Solid Edge part; units mm, degrees
sketch "Sketch1" plane through (0, 0, 0) normal (1, 0, 0) x (0, 1, 0)
  line L0 (0, 0) -> (0, 3.175)
  line L1 (22.225, 3.175) -> (0, 3.175)
  line L2 (22.225, 25.4) -> (22.225, 3.175)
  line L3 (22.225, 25.4) -> (25.4, 25.4)
  line L4 (25.4, 25.4) -> (25.4, 0)
  line L5 (25.4, 0) -> (0, 0)
  dimension "D1" = 25.4
  dimension "D2" = 25.4
extrude "Protrusion1" add sketch "Sketch1" along normal blind 50.8
sketch "Sketch2" plane through (25.4, 12.7, 0) normal (0, 0, -1) x (-1, 0, 0)
  line L0 (-22.225, -1.778) -> (-22.225, 7.874)
  line L1 (-22.225, 7.874) -> (22.225, 7.874)
  line L2 (22.225, 7.874) -> (22.225, -1.778)
  line L3 (22.225, -1.778) -> (-22.225, -1.778)
  dimension "D1" = 22.225
extrude "Cutout1" cut sketch "Sketch2" against normal through all
fillet "Round_1" radius 3.175 4 edges at (3.175, 10.922, 1.5875) (47.625, 10.922, 1.5875) (47.625, 20.574, 1.5875) (3.175, 20.574, 1.5875)
sketch "Sketch3" plane through (25.4, 25.4, 12.7) normal (0, 1, 0) x (1, 0, 0)
  line L0 (-25.4, -12.7) -> (-25.4, 0)
  line L1 (-25.4, 0) -> (25.4, 0)
  line L2 (25.4, 0) -> (25.4, -12.7)
  line L3 (25.4, -12.7) -> (-25.4, -12.7)
  dimension "D1" = 25.4
extrude "Cutout2" cut sketch "Sketch3" against normal through all
hole "Hole_1" at (42.8625, 25.4, 6.35) direction (0, -1, 0) diameter 3.9675 end up to next
hole "Hole1" at (7.9375, 25.4, 6.35) direction (0, -1, 0) diameter 3.9675 end up to next
sketch "Sketch4" plane through (25.4, 12.7, 0) normal (0, 0, -1) x (-1, 0, 0)
  line L0 (-25.4, -12.7) -> (-25.4, -4.953)
  line L1 (-25.4, -4.953) -> (25.4, -4.953)
  line L2 (25.4, -4.953) -> (25.4, -12.7)
  line L3 (25.4, -12.7) -> (-25.4, -12.7)
  dimension "D1" = 25.4
extrude "Cutout3" cut sketch "Sketch4" against normal through all
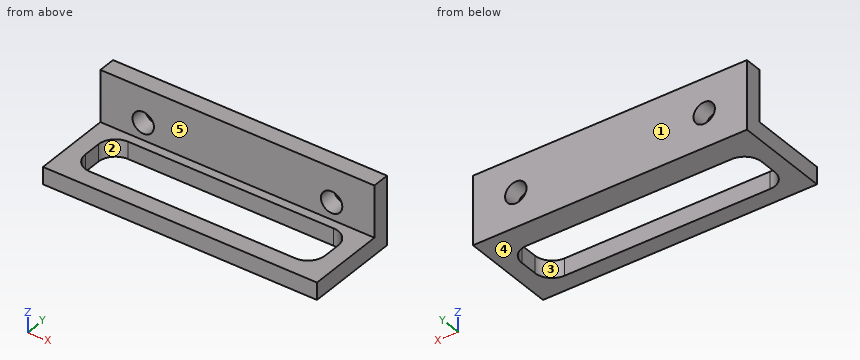
Work out the finished part from the listing and answer in its coordinate system (mm). Face numbers are marked on the shaded views. A direction names the side the tool comes from. Round coordinates to 2 decimals unless told otherwise and drop trailing zeros. Write each loop counter-clockwise with the first axis right and the second up, starting at its lowest first coordinate (ties: lowest second). Pieces come first, ordered by that corner, then holes. Notation, with made-up numbers: (59, 65) - (100, 65) arc R22 cw to (100, 74) - close; hole circle Ø7 at (72.5, -35.5). An arc over 180 degrees is marked (long way). Answer in a Markdown table with one row per item. Add a question column.
1. A cutting plane is placed at B-B, the plane x = 33. Determine the outline of the cut face in (y, z) (3 decimals), and give its area (3 significant figures).
2. A cutting plane is placed at D-D, the plane z = 1.5. Determine the outline of the cut face in (x, y) (3 decimals).
3. A cutting plane is placed at A-A, the plane y = 14.75. Determine the outline of the cut face in (x, z) (3 decimals).
4. The mould has two halves that part along X. Classify the marked faces 1, 2 and 3: +X half, -X half, draft (parallel to the pull), parting line (faces both ways), or undercut.
5. Find the intervals of material crossed by line 1 along X through (y, z) = (23.65, 6.35); line 2 along Z through (x, y) = (46.5, 21.5) (3 decimals); line 3 along Y through (x, z) = (28, 1), in increasing order. Write a range as from..to.
6. Given pin 1 (5 mm diameter, centred on x = 21, z = 10, fed in from -Y) (3 decimals); pin 2 (4 mm diameter, centred on x = 30.5, y = 11, fed in from +Z) (3 decimals); pin 3 (3 mm diameter, centred on x = 42.86, z = 6.35, fed in from -Y), each flat-ended and moving along its own axis, determine where each tip first touches the part or whether it passes through.
7. For the marked faces 4 and 5, determine the directions among +Z, -Z, +X, -X, +Y, -Y from which every point of the face is accessible in a straight line to the end or side of a thin tool.
8. A cutting plane is placed at C-C, the plane z = 6.35. Determine the outline of the cut face in (x, y) (3 decimals), and give its area (3 significant figures).
Worked out:
| question | item | result |
|---|---|---|
| 1 | outline | (7.747, 0) - (10.922, 0) - (10.922, 3.175) - (7.747, 3.175) - close; (20.574, 0) - (25.4, 0) - (25.4, 12.7) - (22.225, 12.7) - (22.225, 3.175) - (20.574, 3.175) - close |
| 1 | area | 55.6 mm^2 |
| 2 | outline | (0, 7.747) - (50.8, 7.747) - (50.8, 25.4) - (0, 25.4) - close; hole (3.175, 14.097) arc R3.175 ccw to (6.35, 10.922) - (44.45, 10.922) arc R3.175 ccw to (47.625, 14.097) - (47.625, 17.399) arc R3.175 ccw to (44.45, 20.574) - (6.35, 20.574) arc R3.175 ccw to (3.175, 17.399) - close |
| 3 | outline | (0, 0) - (3.175, 0) - (3.175, 3.175) - (0, 3.175) - close; (47.625, 0) - (50.8, 0) - (50.8, 3.175) - (47.625, 3.175) - close |
| 4 | face 1 | draft |
| 4 | face 2 | undercut |
| 4 | face 3 | undercut |
| 5 | line 1 | 0..5.95, 9.92..40.88, 44.85..50.8 |
| 5 | line 2 | 0..3.175 |
| 5 | line 3 | 7.75..10.92, 20.57..25.4 |
| 6 | pin 1 | y = 22.225 |
| 6 | pin 2 | z = 3.175 |
| 6 | pin 3 | through |
| 7 | face 4 | -Z, +X, -X, +Y, -Y |
| 7 | face 5 | +Z, +X, -X, -Y |
| 8 | outline | (0, 22.225) - (5.954, 22.225) - (5.954, 25.4) - (0, 25.4) - close; (9.921, 22.225) - (40.879, 22.225) - (40.879, 25.4) - (9.921, 25.4) - close; (44.846, 22.225) - (50.8, 22.225) - (50.8, 25.4) - (44.846, 25.4) - close |
| 8 | area | 136 mm^2 |
